from build123d import *

# Parameters (mm, degrees)
SKETCH1_R           = 45.847
SKETCH1_R_2         = 42.8625
BOSS_EXTRUDE1_DEPTH = 112
CUT_EXTRUDE1_DEPTH  = 4


with BuildPart() as part:
    # Sketch1 → Boss-Extrude1 (new body)
    with BuildSketch(Plane.XY):
        Circle(SKETCH1_R)
        Circle(SKETCH1_R_2, mode=Mode.SUBTRACT)
    extrude(amount=BOSS_EXTRUDE1_DEPTH)

    # Sketch3 → Cut-Extrude1 (cut)
    with BuildSketch(Plane(origin=(0, 0, 0), x_dir=(-1, 0, 0), z_dir=(0, 0, -1))):
        Polygon((6, 45.847), (-6, 45.847), (-6, 6), (-45.847, 6), (-45.847, -6), (-6, -6), (-6, -45.847), (6, -45.847), (6, -6), (45.847, -6), (45.847, 6), (6, 6), align=None)
    extrude(amount=-CUT_EXTRUDE1_DEPTH, mode=Mode.SUBTRACT)


solid = part.part
Here's how the part is built. I have some questions about the finished solid (model axes, mm). A direction names the side the tool comes from. Give positions to 0.01 mm unless a question says otherwise; leave off trailing zeros. Order: outer loops, then holes, each group sorted by start corner. A loop starts at its lowest first (then second) coordinate and runs counter-clockwise, first axis right, second up. Notation, with made-up numbers: (55, -26.5) -> (93, -26.5) arc R24 cw to (93, -16.5) -> close; hole circle Ø5 at (89.5, -16). An arc over 180 degrees is marked (long way). One line per item, written item: value. Start each with the question number.
1. Imagine slicing it at C-C, the plane z = 93. List the corners of the cut face in (x, y) for me (1 decimal).
2. I need wall thicknesses on probe 1 along Y at (x, z) = (0, 59.5); probe 2 along X at (y, z) = (1, 22); probe 3 along Y at (x, z) = (-31.5, 66). Which ranges of each line are inside material? Lowest first, please. Write a range as from..to.
3. For faces 1 (the face through (44, 6, 2)), 2 (the face through (6, 44, 2)), 3 (the face through (23.043, 36.142, 55.216)), which set-ups out of +Z, -Z, +X, -X, +Y, -Y let a thin tool reach every point of the face, with its end or its side?
4. Imagine slicing it at A-A, the plane y = 0. List the corners of the cut face in (x, z) for me.
5. We'd pull the mould along Y, two halves only. Please class faces 4 (the face through (-6, 44, 2)), 5 (the face through (-44, 0, 4)), 6 (the face through (-5.968, 45.457, 55.216)): released by +Y, released by -Y, zero draft, split by the parting line, or undercut.
6. Will these pins go through, and if not, where does the flat tip stop? pin 1 Ø3 at (x, z) = (25.5, 71) entering from -Y; pin 2 Ø6 at (y, z) = (-19.5, 89) entering from -X; pin 3 Ø1 at (x, z) = (15, 52) entering from +Y.
Values follow:
1. outline: circle Ø91.7 at (0, 0); hole circle Ø85.7 at (0, 0)
2. probe 1: y = -45.85..-42.86, 42.86..45.85
2. probe 2: x = -45.84..-42.85, 42.85..45.84
2. probe 3: y = -33.31..-29.07, 29.07..33.31
3. face 1: -Z, +X, -X
3. face 2: -Z, +Y, -Y
3. face 3: +Z, -Z
4. outline: (-45.85, 4) -> (-42.86, 4) -> (-42.86, 112) -> (-45.85, 112) -> close; (42.86, 4) -> (45.85, 4) -> (45.85, 112) -> (42.86, 112) -> close
5. face 4: zero draft
5. face 5: undercut
5. face 6: split by the parting line
6. pin 1: stops at y = -39.06
6. pin 2: stops at x = -42.77
6. pin 3: stops at y = 43.49
